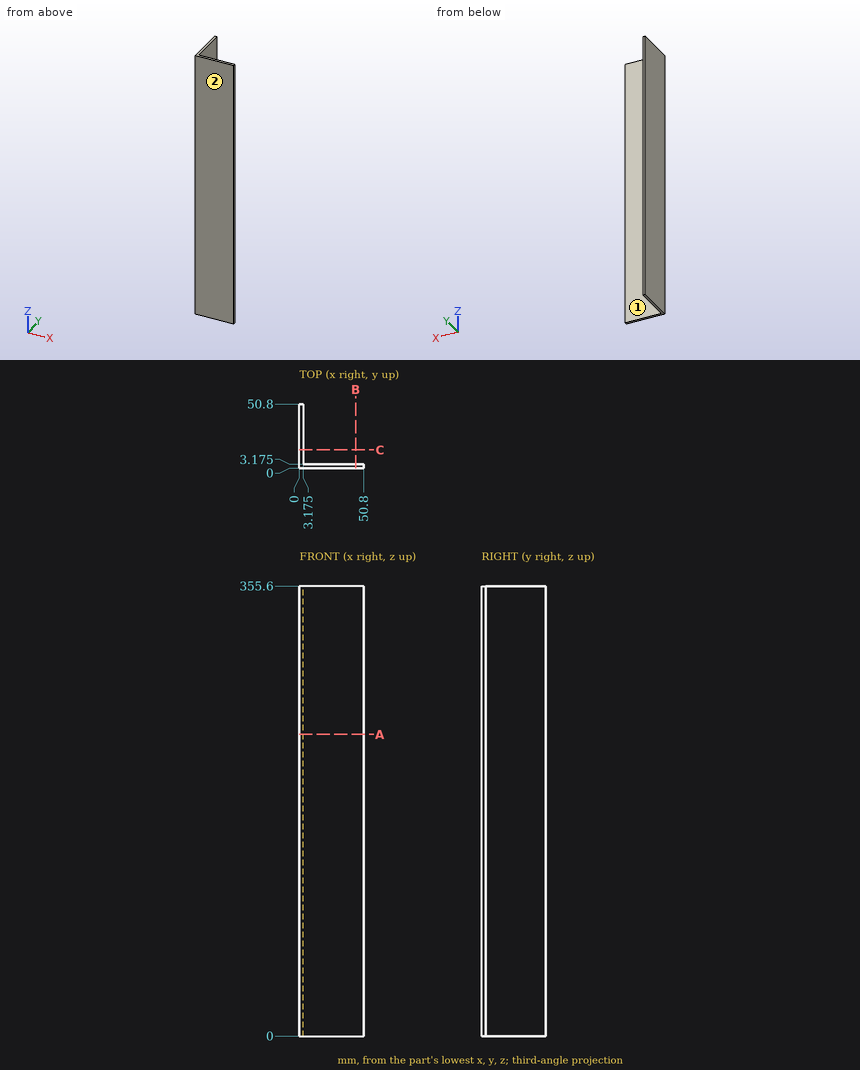
Geometry check sheet. Reference: drawing and pictorial views, mm from the part's lowest x, y, z. A direction names the side the tool comes from. Coordinates: 2 decimals unless noted, no trailing zeros. Order: outer loops, then holes, each group sorted by start corner. A loop starts at its lowest first (then second) coordinate and runs counter-clockwise, first axis right, second up. Notation, with made-up numbers: (21, -11) - (40, -11) arc R18 cw to (40, -1) - close; hole circle Ø1 at (-10, 22). An arc over 180 degrees is marked (long way). One line per item, written item: value.
(1) Depth check by flat-ended pin: pin 1 Ø1 at (y, z) = (22, 197) entering from +X (3 decimals); pin 2 Ø1 at (x, z) = (25.5, 198.5) entering from -Y; pin 3 Ø5 at (x, z) = (11, 222) entering from +Y (3 decimals). Enter the tip coordinate at first touch or a pass-through.
Data:
pin 1: stops at x = 3.175
pin 2: stops at y = 0
pin 3: stops at y = 3.175
(2) Sectioned sample at B-B (x = 44.5). Enter the section's corners in (y, z) (3 decimals), and give its area (3 significant figures).
Data:
outline: (0, 0) - (3.175, 0) - (3.175, 355.6) - (0, 355.6) - close
area: 1,130 mm^2
(3) Thickness scan on probe 1 along Y at (x, z) = (13.5, 189) (3 decimals). Record the ranges inside material, lowest first. Write a range as from..to.
Data:
probe 1: y = 0..3.175
(4) Access from +Z, -Z, +X, -X, +Y, -Y to the whole of each face (thin tool, end or side, straight path). Record for the marked faces 1 and 2.
Data:
face 1: +Z, -Z, +X, +Y
face 2: +Z, -Z, +X, -X, -Y
(5) Sectioned sample at A-A (z = 238.5). Enter the section's corners in (x, y) (3 decimals).
Data:
outline: (0, 0) - (50.8, 0) - (50.8, 3.175) - (3.175, 3.175) - (3.175, 50.8) - (0, 50.8) - close
